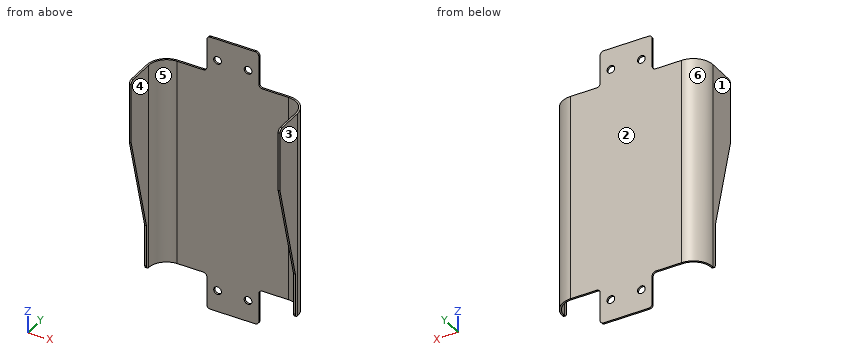
```python
from build123d import *

# Parameters (mm, degrees)
BOSS_EXTRUDE1_DEPTH = 116
SKETCH2_W           = 29
SKETCH2_H           = 20
BOSS_EXTRUDE2_DEPTH = 1
CUT_EXTRUDE1_DEPTH  = 163.549223314
FILLET1_R           = 2
SKETCH4_R           = 2.15
CUT_EXTRUDE2_DEPTH  = 1


with BuildPart() as part:
    # Sketch1 → Boss-Extrude1 (new body)
    with BuildSketch(Plane.XY):
        with BuildLine():
            Line((42, -18.5), (42, 18.5))
            ThreePointArc((42, 18.5), (38.778174593, 26.278174593), (31, 29.5))
            Line((31, 29.5), (-31, 29.5))
            ThreePointArc((-31, 29.5), (-38.778174593, 26.278174593), (-42, 18.5))
            Line((-42, 18.5), (-42, -18.5))
            ThreePointArc((-42, -18.5), (-38.778174593, -26.278174593), (-31, -29.5))
            Line((-31, -29.5), (31, -29.5))
            ThreePointArc((31, -29.5), (38.778174593, -26.278174593), (42, -18.5))
        make_face()
        with BuildLine():
            ThreePointArc((-41, -18.5), (-38.071067812, -25.571067812), (-31, -28.5))
            Line((-31, -28.5), (31, -28.5))
            ThreePointArc((31, -28.5), (38.071067812, -25.571067812), (41, -18.5))
            Line((41, -18.5), (41, 18.5))
            ThreePointArc((41, 18.5), (38.071067812, 25.571067812), (31, 28.5))
            Line((31, 28.5), (-31, 28.5))
            ThreePointArc((-31, 28.5), (-38.071067812, 25.571067812), (-41, 18.5))
            Line((-41, 18.5), (-41, -18.5))
        make_face(mode=Mode.SUBTRACT)
    extrude(amount=-BOSS_EXTRUDE1_DEPTH)

    # Sketch2 → Boss-Extrude2 (add)
    with BuildSketch(Plane(origin=(0, 29.5, 0), x_dir=(1, 0, 0), z_dir=(0, 1, 0))):
        with Locations((0, -10)):
            Rectangle(SKETCH2_W, SKETCH2_H)
        with Locations((0, 126)):
            Rectangle(SKETCH2_W, SKETCH2_H)
    extrude(amount=-BOSS_EXTRUDE2_DEPTH)

    # Sketch3 → Cut-Extrude1 (cut, through all)
    with BuildSketch(Plane(origin=(42, 0, 0), x_dir=(0, 0, -1), z_dir=(1, 0, 0))):
        Polygon((0, 2), (35, 2), (91, 16.5), (116, 16.5), (116, -29.5), (0, -29.5), align=None)
    extrude(amount=-CUT_EXTRUDE1_DEPTH, mode=Mode.SUBTRACT)

    # Fillet1
    fillet1_edges = [part.edges().sort_by_distance(p)[0] for p in [
        (-41.5, 16.5, -116),
        (-14.5, 29, -136),
        (-14.5, 29, -116),
        (14.5, 29, -116),
        (14.5, 29, -136),
        (41.5, 16.5, -116),
        (-14.5, 29, 20),
        (14.5, 29, 20),
        (-14.5, 29, 0),
        (-41.5, 2, 0),
        (14.5, 29, 0),
        (41.5, 2, 0),
    ]]
    fillet(fillet1_edges, radius=FILLET1_R)

    # Sketch4 → Cut-Extrude2 (cut)
    with BuildSketch(Plane(origin=(0, 29.5, 0), x_dir=(1, 0, 0), z_dir=(0, 1, 0))):
        with Locations(Location((8.5, 124, 0), (0, 0, 180))):
            Circle(SKETCH4_R)
        with Locations(Location((-8.5, 124, 0), (0, 0, 180))):
            Circle(SKETCH4_R)
        with Locations(Location((8.5, -8, 0), (0, 0, 180))):
            Circle(SKETCH4_R)
        with Locations(Location((-8.5, -8, 0), (0, 0, 180))):
            Circle(SKETCH4_R)
    extrude(amount=-CUT_EXTRUDE2_DEPTH, mode=Mode.SUBTRACT)


solid = part.part
```
Geometry: final body of the model. Coordinates: model frame, mm. Face numbers are marked on the shaded views. A direction names the side the tool comes from. Round coordinates to 2 decimals unless told otherwise and drop trailing zeros. Order: outer loops, then holes, each group sorted by start corner. A loop starts at its lowest first (then second) coordinate and runs counter-clockwise, first axis right, second up. Notation, with made-up numbers: (-34.5, 52) -> (-18.5, 52) arc R18 ccw to (-18.5, 79) -> close; hole circle Ø6 at (-38.5, 33). An arc over 180 degrees is marked (long way). Use one line per item in the form item = value.
(1) Access query for the marked faces 5 and 6. Directions: +Z, -Z, +X, -X, +Y, -Y. A direction counts if a zero-diameter tool reaches every point of the face in a straight line with its end or side. Return the directions, or none.
Results list:
face_5 = +Z, -Z, -Y
face_6 = +Z, -Z, -X, +Y
(2) First-contact query: pin 1 Ø3 at (y, z) = (23.5, -40) entering from +X; pin 2 Ø10 at (y, z) = (25, -99.5) entering from +X; pin 3 Ø0.5 at (y, z) = (29, -123.5) entering from -X. Flat tips, straight axial feed; report the tip coordinate or a pass-through.
Results list:
pin_1 = 41.43
pin_2 = 41.9
pin_3 = -14.5
(3) Ray query, probe 1 along Z at (x, y) = (8.5, 29.2); probe 2 along X at (y, z) = (15, -78.5); probe 3 along Y at (x, z) = (3.5, -10.5). Return the intervals inside material, ascending. Write a range as [from, to].
Results list:
probe_1 = [-136, -126.15], [-121.85, 5.85], [10.15, 20]
probe_2 = [-42, -41], [41, 42]
probe_3 = [28.5, 29.5]
(4) Section C-C on y = 23.5. Return loops of the section in (x, z), and give its area (3 significant figures).
Results list:
outline = (-40.8, -116) -> (-39.66, -116) -> (-39.66, 0) -> (-40.8, 0) -> close; (39.66, -116) -> (40.8, -116) -> (40.8, 0) -> (39.66, 0) -> close
area = 264 mm^2
(5) Draft query along X for the marked faces 1, 2, 3 and 4. Return one class per face: pulls with the +X half, pulls with the -X half, needs draft (parallel to the pull), parting line crosses it, or undercut.
Results list:
face_1 = pulls with the -X half
face_2 = needs draft
face_3 = pulls with the +X half
face_4 = undercut
(6) Section D-D on z = -10.5. Return loops of the section in (x, y).
Results list:
outline = (-42, 2) -> (-41, 2) -> (-41, 18.5) arc R10 cw to (-31, 28.5) -> (31, 28.5) arc R10 cw to (41, 18.5) -> (41, 2) -> (42, 2) -> (42, 18.5) arc R11 ccw to (31, 29.5) -> (-31, 29.5) arc R11 ccw to (-42, 18.5) -> close
(7) Section A-A on z = 8. Return loops of the section in (x, y).
Results list:
outline = (-14.5, 28.5) -> (-10.65, 28.5) -> (-10.65, 29.5) -> (-14.5, 29.5) -> close; (-6.35, 28.5) -> (6.35, 28.5) -> (6.35, 29.5) -> (-6.35, 29.5) -> close; (10.65, 28.5) -> (14.5, 28.5) -> (14.5, 29.5) -> (10.65, 29.5) -> close
(8) Section B-B on x = 8.5. Return loops of the section in (y, z).
Results list:
outline = (28.5, -136) -> (29.5, -136) -> (29.5, -126.15) -> (28.5, -126.15) -> close; (28.5, -121.85) -> (29.5, -121.85) -> (29.5, 5.85) -> (28.5, 5.85) -> close; (28.5, 10.15) -> (29.5, 10.15) -> (29.5, 20) -> (28.5, 20) -> close
